```python
from build123d import *

# Parameters (mm, degrees)
SKETCH2_W            = 66
SKETCH2_H            = 50
BOSS_EXTRUDE1_DEPTH  = 3
SKETCH3_R            = 1.25
CUT_EXTRUDE1_DEPTH   = 3
CUT_EXTRUDE2_DEPTH   = 1.5
CUT_EXTRUDE3_DEPTH   = 42.509035161
BOSS_EXTRUDE2_START  = 1.5
SKETCH6_R            = 3
SKETCH6_R_2          = 1.25
BOSS_EXTRUDE2_DEPTH  = 1.5
FILLET1_R            = 3
BOSS_EXTRUDE3_DEPTH  = 30
FILLET2_R            = 0.5
FILLET2_OF_MIRROR1_R = 0.5


with BuildPart() as part:
    # Sketch2 → Boss-Extrude1 (new body)
    with BuildSketch(Plane.XY):
        Rectangle(SKETCH2_W, SKETCH2_H)
    extrude(amount=BOSS_EXTRUDE1_DEPTH)

    # Sketch3 → Cut-Extrude1 (cut)
    with BuildSketch(Plane.XY.offset(3)):
        with Locations((-30, 22)):
            Circle(SKETCH3_R)
        with Locations((30, 22)):
            Circle(SKETCH3_R)
        with Locations((30, -22)):
            Circle(SKETCH3_R)
        with Locations((-30, -22)):
            Circle(SKETCH3_R)
    extrude(amount=-CUT_EXTRUDE1_DEPTH, mode=Mode.SUBTRACT)

    # Sketch4 → Cut-Extrude2 (cut)
    with BuildSketch(Plane(origin=(0, 0, 0), x_dir=(-1, 0, 0), z_dir=(0, 0, -1))):
        Polygon((30, 24.424871131), (32.1, 23.212435565), (32.1, 20.787564435), (30, 19.575128869), (27.9, 20.787564435), (27.9, 23.212435565), align=None)
        Polygon((-30, 24.424871131), (-27.9, 23.212435565), (-27.9, 20.787564435), (-30, 19.575128869), (-32.1, 20.787564435), (-32.1, 23.212435565), align=None)
        Polygon((-30, -19.575128869), (-27.9, -20.787564435), (-27.9, -23.212435565), (-30, -24.424871131), (-32.1, -23.212435565), (-32.1, -20.787564435), align=None)
        Polygon((30, -19.575128869), (32.1, -20.787564435), (32.1, -23.212435565), (30, -24.424871131), (27.9, -23.212435565), (27.9, -20.787564435), align=None)
    extrude(amount=-CUT_EXTRUDE2_DEPTH, mode=Mode.SUBTRACT)

    # Sketch5 → Cut-Extrude3 (cut, through all)
    with BuildSketch(Plane(origin=(0, 0, 0), x_dir=(-1, 0, 0), z_dir=(0, 0, -1))):
        Polygon((-1.5, 1.120014204), (-1.5, 19), (-27, 19), (-27, -6.435541351), align=None)
        Polygon((27, 19), (1.5, 19), (1.5, 1.120014204), (27, -6.435541351), align=None)
        Polygon((0, -1.564458649), (-27, -9.564458649), (-27, -19), (27, -19), (27, -9.564458649), align=None)
    extrude(amount=-CUT_EXTRUDE3_DEPTH, mode=Mode.SUBTRACT)

    # Sketch6 → Boss-Extrude2 (add)
    # profile 1 of 4: a face of its own
    with BuildSketch(Plane.XY.offset(3).offset(BOSS_EXTRUDE2_START)):
        with Locations((30, 22)):
            Circle(SKETCH6_R)
        with Locations((30, 22)):
            Circle(SKETCH6_R_2, mode=Mode.SUBTRACT)
    # profile 2 of 4: a face of its own
    with BuildSketch(Plane.XY.offset(3).offset(BOSS_EXTRUDE2_START)):
        with Locations(Location((-30, 22, 0), (0, 0, 180))):
            Circle(SKETCH6_R)
        with Locations((-30, 22)):
            Circle(SKETCH6_R_2, mode=Mode.SUBTRACT)
    # profile 3 of 4: a face of its own
    with BuildSketch(Plane.XY.offset(3).offset(BOSS_EXTRUDE2_START)):
        with Locations(Location((-30, -22, 0), (0, 0, 180))):
            Circle(SKETCH6_R)
        with Locations((-30, -22)):
            Circle(SKETCH6_R_2, mode=Mode.SUBTRACT)
    # profile 4 of 4: a face of its own
    with BuildSketch(Plane.XY.offset(3).offset(BOSS_EXTRUDE2_START)):
        with Locations((30, -22)):
            Circle(SKETCH6_R)
        with Locations((30, -22)):
            Circle(SKETCH6_R_2, mode=Mode.SUBTRACT)
    extrude(amount=-BOSS_EXTRUDE2_DEPTH)

    # Fillet1
    fillet1_edges = [part.edges().sort_by_distance(p)[0] for p in [
        (27, -9.564458649, 1.5),
        (-27, -9.564458649, 1.5),
        (-27, -6.435541351, 1.5),
        (27, -6.435541351, 1.5),
        (0, -1.564458649, 1.5),
        (1.5, 1.120014204, 1.5),
        (-1.5, 1.120014204, 1.5),
        (1.5, 19, 1.5),
        (-1.5, 19, 1.5),
        (-33, 25, 1.5),
        (-33, -25, 1.5),
        (33, -25, 1.5),
        (33, 25, 1.5),
    ]]
    fillet(fillet1_edges, radius=FILLET1_R - 0.0001)  # a hair under: the kernel refuses the full size

    # Sketch7 → Boss-Extrude3 (add, symmetric)
    with BuildSketch(Plane(origin=(0, 0, 0), x_dir=(0, 0, -1), z_dir=(1, 0, 0))):
        Polygon((0, 25), (0, 27.5), (-4, 27.5), (-3, 25), align=None)
    boss_extrude3 = extrude(amount=BOSS_EXTRUDE3_DEPTH, both=True)

    # Fillet2
    fillet2_edges = [part.edges().sort_by_distance(p)[0] for p in [
        (0, 27.5, 4),
    ]]
    fillet(fillet2_edges, radius=FILLET2_R)

    # Mirror1: Boss-Extrude3 across plane
    add(boss_extrude3.mirror(Plane.ZX))

    # Fillet2 of Mirror1
    fillet2_of_mirror1_edges = [part.edges().sort_by_distance(p)[0] for p in [
        (0, -27.5, 4),
    ]]
    fillet(fillet2_of_mirror1_edges, radius=FILLET2_OF_MIRROR1_R)


solid = part.part
```
The listing builds one solid part. Answer for the finished solid, in the listing's coordinates (mm). A direction names the side the tool comes from. Give positions to 0.01 mm unless a question says otherwise; leave off trailing zeros. Order: outer loops, then holes, each group sorted by start corner. A loop starts at its lowest first (then second) coordinate and runs counter-clockwise, first axis right, second up. Notation, with made-up numbers: (67, -12.75) -> (96, -12.75) arc R19 cw to (96, 2.25) -> close; hole circle Ø6 at (9.5, -25.5). An arc over 180 degrees is marked (long way). One line per item, written item: value.
1) Find section B-B, the plane x = 6.5. Determine the outline of the cut face in (y, z).
Reported:
outline: (-27.5, 0) -> (-19, 0) -> (-19, 3) -> (-25, 3) -> (-26.81, 3.73) arc R0.5 ccw to (-27.5, 3.26) -> close; (-3.49, 0) -> (-0.36, 0) -> (-0.36, 3) -> (-3.49, 3) -> close; (19, 0) -> (27.5, 0) -> (27.5, 3.26) arc R0.5 ccw to (26.81, 3.73) -> (25, 3) -> (19, 3) -> close
2) A tool of negligible diameter and unlimited length cuts with its end or side. For faces 1 (the cylindrical face through (2.08, 1.59, 1.52)), 2 (the cylindrical face through (27, 22, 4)), 3 (the flat face through (31.035, -23.827, 0.74)), from which of +Z, -Z, +X, -X, +Y, -Y can it reach the whole face along a straight path? Write none if from no direction.
Reported:
face 1: +Z, -Z
face 2: +Z
face 3: -Z
3) Determine the mould class of faces 4 (the flat face through (31, -23, 4.5)), 5 (the cylindrical face through (-26.42, -10.03, 1.52)) for opening direction Z: pulls with the +Z half, pulls with the -Z half, needs draft (parallel to the pull), parting line crosses it, or undercut.
Reported:
face 4: pulls with the +Z half
face 5: needs draft
4) Find section C-C, the plane z = 0.8. Count the separate pieces of the cut face and the enclosed holes in it, plus the area to 3 significant figures.
Reported:
separate pieces: 1
enclosed holes: 7
area: 1,720 mm^2
5) Flat-ended cylindrical pins translate along their axes: P1, Ø1.5, axis at x = -1, y = -21.5, coming from the +Z side; P2, Ø1, axis at x = -11, y = -5.5, coming from the +Z side; P3, Ø2, axis at y = -26.5, z = 1, coming from the -X side; P4, Ø1, axis at x = 22, z = 4, coming from the +Y side. Find the tip coordinate at first contact, or state that the pin passes through.
Reported:
P1: stops at z = 3
P2: passes through
P3: stops at x = -30
P4: stops at y = 27.44
6) Find section D-D, the plane y = 17.5. Determine the outline of the cut face in (x, z), plus the area to 3 significant figures.
Reported:
outline: (-33, 0) -> (-27, 0) -> (-27, 3) -> (-33, 3) -> close; (-1.9, 0) -> (1.9, 0) -> (1.9, 3) -> (-1.9, 3) -> close; (27, 0) -> (33, 0) -> (33, 3) -> (27, 3) -> close
area: 47.4 mm^2
7) Find section A-A, the plane y = -15.5. Determine the outline of the cut face in (x, z), plus the area to 3 significant figures.
Reported:
outline: (-33, 0) -> (-27, 0) -> (-27, 3) -> (-33, 3) -> close; (27, 0) -> (33, 0) -> (33, 3) -> (27, 3) -> close
area: 36.0 mm^2
8) Find the intervals of material crossed by line 1 (X direction, y = 10, z = 2.45); line 2 (Y direction, x = -12, z = 0.6); line 3 (Y direction, x = -22.5, z = 2), in increasing order.
Reported:
line 1: x = -33 to -27, -1.5 to 1.5, 27 to 33
line 2: y = -27.5 to -19, -5.12 to -1.99, 19 to 27.5
line 3: y = -27.5 to -19, -8.23 to -5.1, 19 to 27.5
